from build123d import *

# Parameters (mm, degrees)
SKETCH1_R                = 4.755
BOSS_EXTRUDE1_DEPTH      = 33.3
BOSS_EXTRUDE1_DRAFT      = 2.000000000000002
SKETCH2_R                = 4.255
CUT_EXTRUDE1_DEPTH       = 33.3
CUT_EXTRUDE1_DRAFT       = 2.000000000000002
SKETCH3_R                = 7.292967388121313
CUT_EXTRUDE2_DEPTH       = 6.2
SKETCH4_R                = 5.47150877
BOSS_EXTRUDE2_DEPTH      = 6.2
BOSS_EXTRUDE2_TAPER      = 2.000000000000002
SKETCH5_R                = 4.755000000000001
CUT_EXTRUDE3_DEPTH       = 6.2
CUT_EXTRUDE3_DRAFT       = 2.000000000000002
BOSS_EXTRUDE3_DEPTH      = 0.1
BOSS_EXTRUDE3_DEPTH_BACK = 0.5
SKETCH8_R                = 5.47150877
SKETCH8_R_2              = 4.471508770848837
FILLET3_R                = 1
FILLET4_R                = 1
FILLET5_R                = 1
FILLET6_R                = 1
FILLET7_R                = 1


with BuildPart() as part:
    # Sketch1 → Boss-Extrude1 (with draft: the straight prism first)
    with BuildSketch(Plane(origin=(0, 0, 0), x_dir=(1, 0, 0), z_dir=(0, 1, 0))):
        Circle(SKETCH1_R)
    extrude(amount=-BOSS_EXTRUDE1_DEPTH)
    # Boss-Extrude1: the draft: its side faces are tilted about the plane it starts from
    boss_extrude1_sides = [part.faces().sort_by_distance(p)[0] for p in [
        (-4.755, -16.65, 0),
    ]]
    draft(boss_extrude1_sides, Plane(origin=(0, 0, 0), x_dir=(1, 0, 0), z_dir=(0, 1, 0)), BOSS_EXTRUDE1_DRAFT)


with BuildPart() as cut_extrude1_tool:
    # Sketch2 → Cut-Extrude1 (with draft: the straight prism first)
    with BuildSketch(Plane(origin=(0, 0, 0), x_dir=(1, 0, 0), z_dir=(0, 1, 0))):
        Circle(SKETCH2_R)
    extrude(amount=-CUT_EXTRUDE1_DEPTH)
    # Cut-Extrude1: the draft: its side faces are tilted about the plane it starts from
    cut_extrude1_sides = [cut_extrude1_tool.faces().sort_by_distance(p)[0] for p in [
        (-4.255, -16.65, 0),
    ]]
    draft(cut_extrude1_sides, Plane(origin=(0, 0, 0), x_dir=(1, 0, 0), z_dir=(0, 1, 0)), CUT_EXTRUDE1_DRAFT)


with BuildPart() as part_1:
    add(part.part)

    # Cut-Extrude1: cut by cut_extrude1_tool
    add(cut_extrude1_tool.part, mode=Mode.SUBTRACT)

    # Sketch3 → Cut-Extrude2 (cut)
    with BuildSketch(Plane(origin=(0, 0, 0), x_dir=(1, 0, 0), z_dir=(0, 1, 0))):
        Circle(SKETCH3_R)
    extrude(amount=-CUT_EXTRUDE2_DEPTH, mode=Mode.SUBTRACT)

    # Sketch4 → Boss-Extrude2 (add)
    with BuildSketch(Plane(origin=(0, -6.2, 0), x_dir=(1, 0, 0), z_dir=(0, 1, 0))):
        Circle(SKETCH4_R)
    extrude(amount=BOSS_EXTRUDE2_DEPTH, taper=BOSS_EXTRUDE2_TAPER)


with BuildPart() as cut_extrude3_tool:
    # Sketch5 → Cut-Extrude3 (with draft: the straight prism first)
    with BuildSketch(Plane(origin=(0, 0, 0), x_dir=(1, 0, 0), z_dir=(0, 1, 0))):
        Circle(SKETCH5_R)
    extrude(amount=-CUT_EXTRUDE3_DEPTH)
    # Cut-Extrude3: the draft: its side faces are tilted about the plane it starts from
    cut_extrude3_sides = [cut_extrude3_tool.faces().sort_by_distance(p)[0] for p in [
        (-4.755, -3.1, 0),
    ]]
    draft(cut_extrude3_sides, Plane(origin=(0, 0, 0), x_dir=(1, 0, 0), z_dir=(0, 1, 0)), CUT_EXTRUDE3_DRAFT)


with BuildPart() as part_2:
    add(part_1.part)

    # Cut-Extrude3: cut by cut_extrude3_tool
    add(cut_extrude3_tool.part, mode=Mode.SUBTRACT)


with BuildPart() as cut_extrude3_piece_1:
    # of the separate pieces the step leaves, piece 1, a body of its own (cut_extrude3_pieces)
    add(part_2.part.solids().sort_by_distance((5.917861624, -33.3, 0))[0])



with BuildPart() as cut_extrude3_piece_2:
    # of the separate pieces the step leaves, piece 2, a body of its own (cut_extrude3_pieces)
    add(part_2.part.solids().sort_by_distance((5.47150877, -6.2, 0))[0])


with BuildPart() as cut_extrude3_piece_1_1:
    add(cut_extrude3_piece_1.part)

    add(cut_extrude3_piece_2.part)  # Boss-Extrude3 merges Cut-Extrude3 piece 2
    # Sketch8 → Boss-Extrude3 (add, two sides: drawn at the far end of the back side and taken through both)
    with BuildSketch(Plane(origin=(0, -6.2, 0), x_dir=(1, 0, 0), z_dir=(0, 1, 0)).offset(-BOSS_EXTRUDE3_DEPTH_BACK)):
        with Locations(Location((0, 0, 0), (0, 0, 270))):
            Circle(SKETCH8_R)
        with Locations(Location((0, 0, 0), (0, 0, 270))):
            Circle(SKETCH8_R_2, mode=Mode.SUBTRACT)
    extrude(amount=BOSS_EXTRUDE3_DEPTH + BOSS_EXTRUDE3_DEPTH_BACK)

    # Fillet3
    # the kernel refuses this fillet: 1 mm, written as the material it takes off along each edge
    with BuildSketch(Plane(origin=(0, -6.7, 0), x_dir=(-1.8e-16, 0, 1), z_dir=(-1, 0, -1.8e-16))) as fillet3_piece_1:
        with BuildLine():
            CenterArc((5.471508770848837, 0.18605349890898903), FILLET3_R, 180, 10.722559871321096)
            Line((4.488969155594713, 0), (4.471508770848837, 0))
            Line((4.471508770848837, 0), (4.471508770848837, 0.18605349890898903))
        make_face()
    revolve(axis=Axis((0, -6.7, 0), (0, 1, 0)), mode=Mode.SUBTRACT)

    # Fillet4
    # the kernel refuses this fillet: 1 mm, written as the material it adds along each edge
    with BuildSketch(Plane(origin=(0, -6.1000000000000005, 0), x_dir=(1, 0, 0), z_dir=(0, 0, 1))) as fillet4_piece_1:
        with BuildLine():
            CenterArc((3.9378741267887936, 0.8457151214558971), FILLET4_R, 302.2513636377463, 59.748636362253706)
            Line((4.47150877084877, 1.0658e-13), (4.482181463729969, -0.01691430242900882))
            ThreePointArc((4.482181463729969, -0.01691430242900882), (4.719762732374216, -0.01999999999999957), (4.968016693899662, -0.01999999999999957))
            Line((4.968016693899662, -0.01999999999999957), (4.988004510440043, 0.00069798993405001))
            Line((4.988004510440043, 0.00069798993405001), (4.957252770348271, 0.8813126080924478))
            Line((4.957252770348271, 0.8813126080924478), (4.937264953807889, 0.8806146181583978))
        make_face()
    revolve(axis=Axis((0, -6.1000000000000005, 0), (0, 1, 0)))

    # Fillet5
    # the kernel refuses this fillet: 1 mm, written as the material it takes off along each edge
    with BuildSketch(Plane(origin=(0, -6.1000000000000005, 0), x_dir=(-1.8e-16, 0, 1), z_dir=(-1, 0, -1.8e-16))) as fillet5_piece_1:
        with BuildLine():
            CenterArc((5.4715087708488035, -0.4380156830897022), FILLET5_R, 140.06894109758144, 39.931058902420205)
            Line((4.471508770848803, -0.4380156830897315), (4.471508770848837, 0))
            ThreePointArc((4.471508770848837, 0), (4.5960401438617255, 0.09284229423308599), (4.704691448818901, 0.20384971918314942))
        make_face()
    revolve(axis=Axis((0, -6.1000000000000005, 0), (0, 1, 0)), revolution_arc=90.00000000000001, mode=Mode.SUBTRACT)
    with BuildSketch(Plane(origin=(0, -6.1000000000000005, 0), x_dir=(1, 0, 2e-17), z_dir=(-2e-17, 0, 1))) as fillet5_piece_2:
        with BuildLine():
            CenterArc((5.4715087708488035, -0.4380156830897022), FILLET5_R, 140.06894109758142, 39.931058902420205)
            Line((4.4715087708488035, -0.4380156830897306), (4.471508770848837, 0))
            ThreePointArc((4.471508770848837, 0), (4.596040143861726, 0.09284229423308688), (4.7046914488189016, 0.20384971918314942))
        make_face()
    revolve(axis=Axis((0, -6.1000000000000005, 0), (0, 1, 0)), revolution_arc=270, mode=Mode.SUBTRACT)

    # Fillet6
    # the kernel refuses this fillet: 1 mm, written as the material it adds along each edge
    with BuildSketch(Plane(origin=(0, -6.7, 0), x_dir=(1, 0, 0), z_dir=(0, 0, 1))) as fillet6_piece_1:
        with BuildLine():
            CenterArc((6.018805247042198, -0.8369388067342642), FILLET6_R, 123.18173696935794, 58.818263030642015)
            Line((5.019414420023102, -0.8718383034367649), (4.99942660348272, -0.872536293370815))
            Line((4.99942660348272, -0.872536293370815), (4.968981339054329, -0.00069798993405001))
            Line((4.968981339054329, -0.00069798993405001), (4.98896915559471, 0.01999999999999957))
            ThreePointArc((4.98896915559471, 0.01999999999999957), (5.230238962797434, 0.01999999999999957), (5.460562840459316, 0.01673877613443953))
            Line((5.460562840459316, 0.01673877613443953), (5.471508770000157, -2.407e-13))
        make_face()
    revolve(axis=Axis((0, -6.7, 0), (0, 1, 0)))

    # Fillet7
    # the kernel refuses this fillet: 1 mm, written as the material it takes off along each edge
    with BuildSketch(Plane(origin=(0, -6.7, 0), x_dir=(-1.8e-16, 0, 1), z_dir=(-1, 0, -1.8e-16))) as fillet7_piece_1:
        with BuildLine():
            CenterArc((4.471508770000036, 0.4302918795001718), FILLET7_R, 320.68263745440794, 39.31736254559383)
            Line((5.471508770000037, 0.43029187950020287), (5.47150877, 0))
            ThreePointArc((5.47150877, 0), (5.350554662973599, -0.09300254811217279), (5.245157008521018, -0.2033234636169139))
        make_face()
    revolve(axis=Axis((0, -6.7, 0), (0, 1, 0)), revolution_arc=90.00000000000001, mode=Mode.SUBTRACT)
    with BuildSketch(Plane(origin=(0, -6.1000000000000005, 0), x_dir=(-1.8e-16, 0, 1), z_dir=(-1, 0, -1.8e-16))) as fillet7_piece_2:
        with BuildLine():
            CenterArc((4.47150877, -0.08349825924513077), FILLET7_R, 0, 4.789674454393566)
            Line((5.468016693050807, -1.78e-15), (5.47150877, 0))
            Line((5.47150877, 0), (5.47150877, -0.08349825924513077))
        make_face()
    revolve(axis=Axis((0, -6.1000000000000005, 0), (0, 1, 0)), mode=Mode.SUBTRACT)
    with BuildSketch(Plane(origin=(0, -6.7, 0), x_dir=(1, 0, 2e-17), z_dir=(-2e-17, 0, 1))) as fillet7_piece_3:
        with BuildLine():
            CenterArc((4.471508770000037, 0.43029187950017356), FILLET7_R, 320.6826374544079, 39.317362545594)
            Line((5.471508770000037, 0.4302918795002064), (5.47150877, 0))
            ThreePointArc((5.47150877, 0), (5.3505546629736, -0.0930025481121719), (5.245157008521018, -0.203323463616913))
        make_face()
    revolve(axis=Axis((0, -6.7, 0), (0, 1, 0)), revolution_arc=270, mode=Mode.SUBTRACT)


solid = cut_extrude3_piece_1_1.part
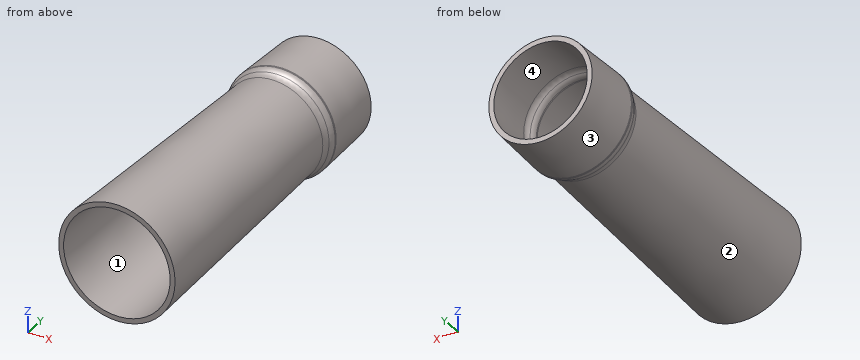
For this review, take the finished solid that the model builds, in its own axes (mm). Face numbers are marked on the shaded views. A direction names the side the tool comes from. Round coordinates to 2 decimals unless told otherwise and drop trailing zeros. Write each loop counter-clockwise with the first axis right and the second up, starting at its lowest first coordinate (ties: lowest second). Pieces come first, ordered by that corner, then holes. Notation, with made-up numbers: (53.25, 72.25) - (106.25, 72.25) arc R28 ccw to (106.25, 96.25) - close; hole circle Ø5 at (53.5, 50.5). An arc over 180 degrees is marked (long way). Use a Markdown table: item, result.
Q1. Wall thickness on line 1 along X through (y, z) = (-2, -4); line 2 along X through (y, z) = (-14, 3); line 3 along Z through (x, y) = (-1.5, -26): over which ranges is each line inside the solid? List them lowest first.
Derived:
| item | result |
|---|---|
| line 1 | x = -3.51 to -2.7, 2.7 to 3.51 |
| line 2 | x = -4.3 to -3.67, 3.67 to 4.3 |
| line 3 | z = -5.46 to -4.94, 4.94 to 5.46 |
Q2. We need section A-A (y = -2.5). Give the boundary of the cut face in (x, z), plus the area to 3 significant figures.
Derived:
| item | result |
|---|---|
| outline | circle Ø10.68 at (0, 0); hole circle Ø9.68 at (0, 0) |
| area | 16.0 mm2 |
Q3. Clearance check with flat-ended pins moving along their axes: pin 1 (2 mm diameter, centred on x = 1.5, z = 2.5, fed in from +Y); pin 2 (5 mm diameter, centred on y = -24.5, z = 0.5, fed in from +X); pin 3 (3 mm diameter, centred on x = 2, y = -21.5, fed in from -Z); pin 4 (3 mm diameter, centred on x = -3, y = -5, fed in from -Z). State where each tip first meets the part, or that it passes through.
Derived:
| item | result |
|---|---|
| pin 1 | passes through |
| pin 2 | stops at x = 5.7 |
| pin 3 | stops at z = -5.49 |
| pin 4 | stops at z = -5.22 |
Q4. The part is to be moulded in two halves that separate along X. For the marked faces 3 and 4, say which applies: pulls with the +X half, pulls with the -X half, needs draft (parallel to the pull), parting line crosses it, or undercut.
Derived:
| item | result |
|---|---|
| face 3 | parting line crosses it |
| face 4 | undercut |
Q5. Machinability: for the marked faces 1 and 2, which of the approach directions +Z, -Z, +X, -X, +Y, -Y give a long, thin tool a straight path to every point of the face, cutting with its end or side? Answer none if there is none.
Derived:
| item | result |
|---|---|
| face 1 | -Y |
| face 2 | none |
